Design review of the part built by this model. Coordinates are the model's own, in mm. A direction names the side the tool comes from. Round coordinates to 2 decimals unless told otherwise and drop trailing zeros. Order: outer loops, then holes, each group sorted by start corner. A loop starts at its lowest first (then second) coordinate and runs counter-clockwise, first axis right, second up. Notation, with made-up numbers: M 24.5,-17.75 L 38.5,-17.75 A9 ccw 38.5,-8.75 Z; hole C 86,21 d3. An arc over 180 degrees is marked long. Use a Markdown table: item, result. Add a question column.
(1) Take a section at B-B (x = 22). Write out the cut boundary in (y, z), then the cut area to 3 significant figures.
(2) Take a section at A-A (z = 40.25). Write out the cut boundary in (x, y).
(3) For pin 1 (1.5 mm diameter, centred on y = 19, z = 21, fed in from +X); pin 2 (9.5 mm diameter, centred on y = 35, z = -27.5, fed in from +X); pin 3 (12 mm diameter, centred on y = 43, z = 2, fed in from -X); pin 4 (2 mm diameter, centred on x = 69, y = 27.5, fed in from +Z), all flat-tipped, find the tip position at first contact; note any pin that passes through.
(4) To check wall thickness, follow probe 1 along X at (y, z) = (0.85, -38.25); probe 2 along X at (y, z) = (1.1, 40.25); probe 3 along Z at (x, y) = (45, 4). State the ranges of each line that lie inside material, in increasing order. Write a range as from..to.
(5) Machinability: for faces 4 (the face through (71, 25, 6.5)), 5 (the face through (78, 25, -12)), 6 (the face through (-62.419, 25.171, 2.683)), 7 (the face through (6, 25, -1.5)), which of the approach directions +Z, -Z, +X, -X, +Y, -Y give a long, thin tool a straight path to every point of the face, cutting with its end or side? Answer none if there is none.
(6) The part is to be moulded in two halves that separate along X. For faces 1 (the face through (-68, 4, -47)), 2 (the face through (-76, 25, -9.5)), 3 (the face through (-58, 25, 6.5)), say which applies: released by +X, released by -X, zero draft, split by the parting line, or undercut.
(7) Take a section at C-C (z = -18.5). Write out the cut boundary in (x, y).
(8) Take a section at D-D (y = 22.5). Count the separate pieces of the cut face and the enclosed holes in it, then the cut area to 3 significant figures.
```python
from build123d import *

# Parameters (mm, degrees)
SKETCH1_W               = 170
SKETCH1_H               = 100
BOSS_EXTRUDE1_DEPTH     = 2
CUT_EXTRUDE7_DEPTH      = 99.635693337
CUT_EXTRUDE7_DEPTH_BACK = 99.635693337
SKETCH14_R              = 2.25
CUT_EXTRUDE8_DEPTH      = 99.635693337
CUT_EXTRUDE8_DEPTH_BACK = 99.635693337
SKETCH15_W              = 54
SKETCH15_H              = 6.5
SKETCH16_R              = 4
SKETCH16_W              = 7
SKETCH16_H              = 6.5
BOSS_EXTRUDE4_DEPTH     = 47
FILLET1_R               = 4
CHAMFER1_SIZE           = 5
FILLET2_R               = 8
SKETCH17_W              = 12.5
SKETCH17_H              = 6.5
BOSS_EXTRUDE5_DEPTH     = 4
CHAMFER2_SIZE           = 4
FILLET3_R               = 12


# Some blends are built 0.0001 mm under size
with BuildPart() as part:
    # Sketch1 → Boss-Extrude1 (new body)
    with BuildSketch(Plane(origin=(0, 0, 0), x_dir=(1, 0, 0), z_dir=(0, 1, 0))):
        Rectangle(SKETCH1_W, SKETCH1_H)
    extrude(amount=BOSS_EXTRUDE1_DEPTH)

    # Sketch14 → Cut-Extrude7 (cut, two sides: drawn at the far end of the back side and taken through both)
    with BuildSketch(Plane(origin=(0, 2, 0), x_dir=(1, 0, 0), z_dir=(0, 1, 0)).offset(-CUT_EXTRUDE7_DEPTH_BACK)):
        with Locations(Location((-40.25, 38.25, 0), (0, 0, 270))):
            Circle(SKETCH14_R)
        with Locations(Location((40.25, 38.25, 0), (0, 0, 270))):
            Circle(SKETCH14_R)
        with Locations(Location((-39.5, -40.25, 0), (0, 0, 270))):
            Circle(SKETCH14_R)
        with Locations(Location((39.5, -40.25, 0), (0, 0, 270))):
            Circle(SKETCH14_R)
    extrude(amount=CUT_EXTRUDE7_DEPTH + CUT_EXTRUDE7_DEPTH_BACK, mode=Mode.SUBTRACT)

    # Sketch15 → Cut-Extrude8 (cut, two sides: drawn at the far end of the back side and taken through both)
    with BuildSketch(Plane(origin=(0, 2, 0), x_dir=(1, 0, 0), z_dir=(0, 1, 0)).offset(-CUT_EXTRUDE8_DEPTH_BACK)):
        with Locations((-30.5, 46.75)):
            Rectangle(SKETCH15_W, SKETCH15_H)
        with Locations((30.5, 46.75)):
            Rectangle(SKETCH15_W, SKETCH15_H)
    extrude(amount=CUT_EXTRUDE8_DEPTH + CUT_EXTRUDE8_DEPTH_BACK, mode=Mode.SUBTRACT)

    # Sketch16 → Boss-Extrude4 (add)
    # profile 1 of 7: a face of its own
    with BuildSketch(Plane(origin=(0, 2, 0), x_dir=(1, 0, 0), z_dir=(0, 1, 0))):
        Polygon((-70, 32.5), (-70, 43.5), (-78, 43.5), (-78, 9.5), (-70, 9.5), align=None)
    # profile 2 of 7: a face of its own
    with BuildSketch(Plane(origin=(0, 2, 0), x_dir=(1, 0, 0), z_dir=(0, 1, 0))):
        Polygon((-57.5, 43.5), (-70, 43.5), (-70, 32.5), (70, 32.5), (70, 43.5), (57.5, 43.5), (3.5, 43.5), (-3.5, 43.5), align=None)
        with Locations(Location((-40.25, 38.25, 0), (0, 0, 270))):
            Circle(SKETCH16_R, mode=Mode.SUBTRACT)
        with Locations(Location((40.25, 38.25, 0), (0, 0, 270))):
            Circle(SKETCH16_R, mode=Mode.SUBTRACT)
    # profile 3 of 7: a face of its own
    with BuildSketch(Plane(origin=(0, 2, 0), x_dir=(1, 0, 0), z_dir=(0, 1, 0))):
        with Locations((0, 46.75)):
            Rectangle(SKETCH16_W, SKETCH16_H)
    # profile 4 of 7: a face of its own
    with BuildSketch(Plane(origin=(0, 2, 0), x_dir=(1, 0, 0), z_dir=(0, 1, 0))):
        Polygon((70, 43.5), (70, 32.5), (70, 9.5), (78, 9.5), (78, 43.5), align=None)
    # profile 5 of 7: a face of its own
    with BuildSketch(Plane(origin=(0, 2, 0), x_dir=(1, 0, 0), z_dir=(0, 1, 0))):
        Polygon((78, 9.5), (70, 9.5), (-56, 9.5), (-56, 1.5), (-55, 1.5), (68, 1.5), (78, 1.5), align=None)
    # profile 6 of 7: a face of its own
    with BuildSketch(Plane(origin=(0, 2, 0), x_dir=(1, 0, 0), z_dir=(0, 1, 0))):
        Polygon((78, -18.5), (78, 1.5), (68, 1.5), (68, -6.5), (73.5, -6.5), (73.5, -9), (68, -9), (68, -18.5), align=None)
    # profile 7 of 7: a face of its own
    with BuildSketch(Plane(origin=(0, 2, 0), x_dir=(1, 0, 0), z_dir=(0, 1, 0))):
        Polygon((-55, 1.5), (-56, 1.5), (-65, 1.5), (-65, -18.5), (-55, -18.5), (-55, -9), (-60.5, -9), (-60.5, -6.5), (-55, -6.5), align=None)
    extrude(amount=BOSS_EXTRUDE4_DEPTH)

    # Fillet1
    fillet1_edges = [part.edges().sort_by_distance(p)[0] for p in [
        (-70, 25.5, -9.5),
        (-56, 25.5, -9.5),
    ]]
    fillet(fillet1_edges, radius=FILLET1_R)

    # Chamfer1
    chamfer1_edges = [part.edges().sort_by_distance(p)[0] for p in [
        (-55, 25.5, -1.5),
        (68, 25.5, -1.5),
    ]]
    chamfer(chamfer1_edges, length=CHAMFER1_SIZE)

    # Fillet2
    fillet2_edges = [part.edges().sort_by_distance(p)[0] for p in [
        (-78, 25.5, -43.5),
        (-65, 25.5, 18.5),
        (78, 25.5, 18.5),
        (78, 25.5, -43.5),
    ]]
    fillet(fillet2_edges, radius=FILLET2_R)

    # Sketch17 → Boss-Extrude5 (add)
    with BuildSketch(Plane(origin=(0, 2, 0), x_dir=(1, 0, 0), z_dir=(0, 1, 0))):
        with Locations((-63.75, 46.75)):
            Rectangle(SKETCH17_W, SKETCH17_H)
        with Locations((63.75, 46.75)):
            Rectangle(SKETCH17_W, SKETCH17_H)
    extrude(amount=BOSS_EXTRUDE5_DEPTH)

    # Chamfer2
    chamfer2_edges = [part.edges().sort_by_distance(p)[0] for p in [
        (70, 6, -46.75),
        (-70, 6, -46.75),
    ]]
    chamfer(chamfer2_edges, length=CHAMFER2_SIZE - 0.0001)  # a hair under: the kernel refuses the full size

    # Fillet3
    # the kernel refuses this fillet: 12 mm, written as the material it takes off along each edge
    with BuildSketch(Plane(origin=(-65, 2, -1.5), x_dir=(0, 0, 1), z_dir=(0, 1, 0))) as fillet3_piece_1:
        with BuildLine():
            CenterArc((11.618950039, 12), FILLET3_R, 194.477512186, 75.522487814)
            Line((0, 9), (0, 0))
            Line((0, 0), (11.618950039, 0))
        make_face()
    extrude(amount=76.047375097, mode=Mode.SUBTRACT)


solid = part.part
```
Verdict:
| question | item | result |
|---|---|---|
| 1 | outline | M 0,-43.5 L 49,-43.5 L 49,-32.5 L 2,-32.5 L 2,-9.5 L 49,-9.5 L 49,-1.5 L 2,-1.5 L 2,50 L 0,50 Z |
| 1 | area | 1,080 mm^2 |
| 2 | outline | M -85,0 L -41.75,0 L -41.75,2 L -85,2 Z; M -37.25,0 L 37.25,0 L 37.25,2 L -37.25,2 Z; M 41.75,0 L 85,0 L 85,2 L 41.75,2 Z |
| 3 | pin 1 | passes through |
| 3 | pin 2 | stops at x = 78 |
| 3 | pin 3 | stops at x = -64.81 |
| 3 | pin 4 | stops at z = 18.5 |
| 4 | probe 1 | x = -85..-42.5, -38..38, 42.5..85 |
| 4 | probe 2 | x = -85..-41.75, -37.25..37.25, 41.75..85 |
| 4 | probe 3 | z = -43.5..-32.5, -9.5..-1.5 |
| 5 | face 4 | +Y |
| 5 | face 5 | +Z, -Z, +X, +Y |
| 5 | face 6 | -X, +Y |
| 5 | face 7 | +Z, +Y |
| 6 | face 1 | released by -X |
| 6 | face 2 | zero draft |
| 6 | face 3 | undercut |
| 7 | outline | M -85,0 L 85,0 L 85,2 L 78,2 L 78,49 L 70,49 L 70,2 L -70,2 L -70,49 L -78,49 L -78,2 L -85,2 Z |
| 8 | separate pieces | 1 |
| 8 | enclosed holes | 2 |
| 8 | area | 3,410 mm^2 |
